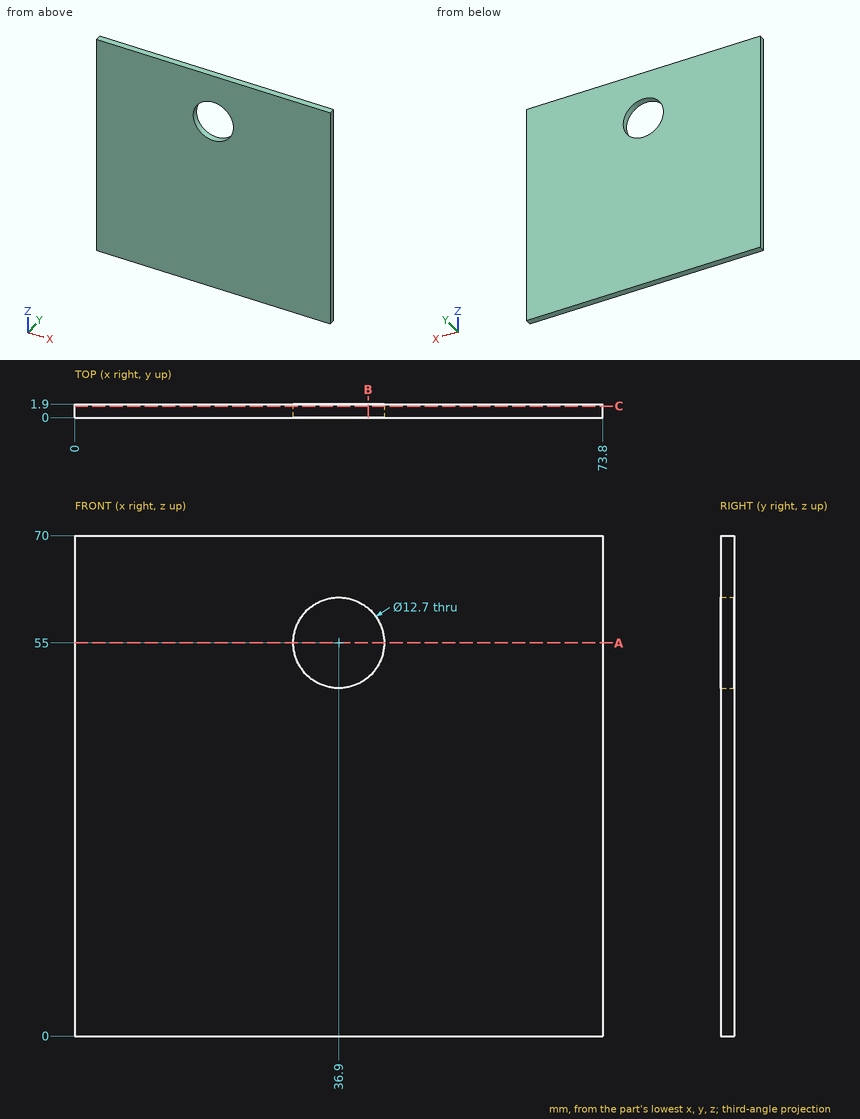
Answer from the drawing. Dimensions are ordinates in mm from the lowest x, y and z of the part. Round coordinates to 2 decimals unless told otherwise and drop trailing zeros. Loops run counter-clockwise (first coordinate to the right, second up) from the corner with the lowest first, then second, coordinate; pieces in that order, holes last.
(1) Each of these flat-tipped pins is pushed along its axis until it touches: P1, Ø10, axis at x = 36.9, z = 55, coming from the -Y side; P2, Ø6, axis at x = 13, z = 54.5, coming from the -Y side. Where does it stop, or does it pass through?
Computed values:
P1: passes through
P2: stops at y = 0
(2) The part is cut by section A-A, the plane z = 55. Give the vertices of the cut face in (x, y).
Computed values:
outline: (0, 0) - (30.55, 0) - (30.55, 1.9) - (0, 1.9) - close; (43.25, 0) - (73.8, 0) - (73.8, 1.9) - (43.25, 1.9) - close
(3) The part is cut by section B-B, the plane x = 41. Give the vertices of the cut face in (y, z), and give its area (3 significant figures).
Computed values:
outline: (0, 0) - (1.9, 0) - (1.9, 50.15) - (0, 50.15) - close; (0, 59.85) - (1.9, 59.85) - (1.9, 70) - (0, 70) - close
area: 115 mm2
(4) The part is cut by section C-C, the plane y = 1.6. Give the vertices of the cut face in (x, z), and give its area (3 significant figures).
Computed values:
outline: (0, 0) - (73.8, 0) - (73.8, 70) - (0, 70) - close; hole circle Ø12.7 at (36.9, 55)
area: 5,040 mm2
(5) Find the intervals of material crossed by L1, parallel to Z at x = 36.9, y = 0.5; L2, parallel to X at y = 0.7, z = 55; L3, parallel to Z at x = 41, y = 1.4, in increasing order.
Computed values:
L1: z = 0 to 48.65, 61.35 to 70
L2: x = 0 to 30.55, 43.25 to 73.8
L3: z = 0 to 50.15, 59.85 to 70
